from build123d import *

# Parameters (mm, degrees)
F0_W     = 139.7
F0_H     = 100.2
F0_R     = 9.525
F0_W_2   = 3.1
F0_H_2   = 1.55
F1_DEPTH = 101.6
F2_DEPTH = 13.7
F4_R     = 9.525
F4_W     = 3.1
F4_H     = 1.55
F5_DEPTH = 13.7
F7_DEPTH = 10


with BuildPart() as f1:
    # F0 (on Front) → F1 (new body)
    with BuildSketch(Plane.XZ):
        with Locations((19.05, -8.02)):
            Rectangle(F0_W, F0_H)
        Circle(F0_R, mode=Mode.SUBTRACT)
        Circle(F0_R)
        Rectangle(F0_W_2, F0_H_2, mode=Mode.SUBTRACT)
        Rectangle(F0_W_2, F0_H_2)
    extrude(amount=F1_DEPTH)

    # F0 (on Front) → F2 (join)
    with BuildSketch(Plane.XZ):
        Circle(F0_R)
        Rectangle(F0_W_2, F0_H_2, mode=Mode.SUBTRACT)
    extrude(amount=-F2_DEPTH)

    # F4 (on offset) → F5 (join)
    with BuildSketch(Plane.XZ.offset(101.6)):
        Circle(F4_R)
        Rectangle(F4_W, F4_H, mode=Mode.SUBTRACT)
    extrude(amount=F5_DEPTH)

    # F6 (on face) → F7 (cut)
    with BuildSketch(Plane(origin=(0, 0, -58.12), x_dir=(1, 0, 0), z_dir=(0, 0, -1))):
        with BuildLine():
            ThreePointArc((21.45, 95.25), (17.3529437252, 96.9470562748), (19.05, 92.85))
            ThreePointArc((19.05, 92.85), (20.7470562748, 93.5529437252), (21.45, 95.25))
        make_face()
        with BuildLine():
            ThreePointArc((21.45, 6.35), (20.7470562748, 8.0470562748), (19.05, 8.75))
            ThreePointArc((19.05, 8.75), (17.3529437252, 4.6529437252), (21.45, 6.35))
        make_face()
    extrude(amount=-F7_DEPTH, mode=Mode.SUBTRACT)


solid = f1.part
Geometry: final body of the model. Coordinates: model frame, mm. A direction names the side the tool comes from. Give positions to 0.01 mm unless a question says otherwise; leave off trailing zeros. Write each loop counter-clockwise with the first axis right and the second up, starting at its lowest first coordinate (ties: lowest second). Pieces come first, ordered by that corner, then holes.
(1) First-contact query: P1, Ø0.5, axis at y = -106, z = 0, coming from the -X side (3 decimals); P2, Ø0.9, axis at x = 0.5, y = 6.5, coming from the +Z side; P3, Ø8, axis at x = 18.5, z = -27.5, coming from the -Y side. Flat tips, straight axial feed; report the tip coordinate or a pass-through.
(2) Cut plane B-B, the plane x = 37.5. Return loops of the section in (y, z), then the cut area to 3 significant figures.
(3) Cut plane A-A, the plane z = 7. Return loops of the section in (x, y).
(4) Access query for faces 1 (the cylindrical face through (-7.559, -108.354, -5.796)), 2 (the flat face through (18, -50, 42.08)), 3 (the flat face through (19, -6, -48.12)). Directions: +Z, -Z, +X, -X, +Y, -Y. A direction counts if a zero-diameter tool reaches every point of the face in a straight line with its end or side. Return the directions, or none.
(5) Cut plane C-C, the plane z = -30.5. Return loops of the section in (x, y), then the cut area to 3 significant figures.
(6) Ray query, line 1 (Y direction, x = 19, z = -52); line 2 (X direction, y = -95.25, z = -52); line 3 (Y direction, x = 34, z = 6.5). Return the intervals inside material, ascending.
(7) Mould query, pull axis X, two halves, no side actions, for faces 4 (the flat face through (19, -95, -48.12)), 5 (the cylindrical face through (-7.559, 6.754, -5.796)), 6 (the flat face through (-50.8, -50, -9)). Classes: released by +X, released by -X, zero draft, split by the parting line, or undercut.
Values follow:
1. P1: stops at x = -9.525
1. P2: stops at z = 9.52
1. P3: stops at y = -101.6
2. outline: (-101.6, -58.12) - (0, -58.12) - (0, 42.08) - (-101.6, 42.08) - close
2. area: 10,200 mm2
3. outline: (-50.8, -101.6) - (-6.46, -101.6) - (-6.46, -115.3) - (6.46, -115.3) - (6.46, -101.6) - (88.9, -101.6) - (88.9, 0) - (6.46, 0) - (6.46, 13.7) - (-6.46, 13.7) - (-6.46, 0) - (-50.8, 0) - close
4. face 1: -Y
4. face 2: +Z, +X, -X, +Y, -Y
4. face 3: -Z
5. outline: (-50.8, -101.6) - (88.9, -101.6) - (88.9, 0) - (-50.8, 0) - close
5. area: 14,200 mm2
6. line 1: y = -101.6 to -97.65, -92.85 to -8.75, -3.95 to 0
6. line 2: x = -50.8 to 16.65, 21.45 to 88.9
6. line 3: y = -101.6 to 0
7. face 4: undercut
7. face 5: split by the parting line
7. face 6: released by -X
